CAD build for the part. Positions are in the model's coordinates, mm. A direction names the side the tool comes from. Give positions to 0.01 mm unless a question says otherwise; leave off trailing zeros. Order: outer loops, then holes, each group sorted by start corner. A loop starts at its lowest first (then second) coordinate and runs counter-clockwise, first axis right, second up.
Solid Edge part; units mm, degrees
sketch "Sketch1" plane through (0, 0, 0) normal (0, 0, 1) x (1, 0, 0)
  circle A0 centre (0, 0) radius 15.748
  circle A1 centre (0, 0) radius 7.62
extrude "Protrusion1" add sketch "Sketch1" along normal blind 7.366
sketch "Sketch2" plane through (0, 0, 0) normal (0, 0, 1) x (1, 0, 0)
  circle A0 centre (0, -11.684) radius 6.858
extrude "ExtrudedCutout_1" cut sketch "Sketch2" along normal blind 6.858
sketch "Sketch3" plane through (0, 0, 7.366) normal (0, 0, 1) x (1, 0, 0)
  circle A0 centre (0, -11.684) radius 3.683
extrude "ExtrudedCutout_3" cut sketch "Sketch3" against normal blind 7.0384
pattern_circular "Pattern1" count 4 over 360 about axis through (0, 0, 7.366) along (0, 0, 1) of "ExtrudedCutout_1", "ExtrudedCutout_3"
sketch "Sketch4" plane through (0, 0, 7.366) normal (0, 0, 1) x (1, 0, 0)
  circle A0 centre (0, 0) radius 7.62
  circle A1 centre (-11.684, 0) radius 3.683
  circle A2 centre (0, 11.684) radius 3.683
  circle A3 centre (11.684, 0) radius 3.683
  circle A4 centre (0, -11.684) radius 3.683
  circle A5 centre (0, 0) radius 15.748
extrude "ExtrudedProtrusion_5" add sketch "Sketch4" along normal blind 9.779
sketch "Sketch5" plane through (0, 0, 17.145) normal (0, 0, 1) x (1, 0, 0)
  circle A0 centre (0, 0) radius 19.2555
extrude "ExtrudedCutout_4" cut sketch "Sketch5" against normal blind 6.35
Item 1: Slice it at C-C (x = 5). Give the cut face in (y, z) (3 decimals).
Item 2: Wall check: L1, parallel to X at y = 0, z = 8; L2, parallel to Y at x = -1.5, z = 9.25. Give the ranges that are in metal, low to high.
Item 3: Slice it at A-A (x = 0). Give the cut face in (y, z) (3 decimals), and give its area (3 significant figures).
Item 4: Tool access for faces 1 (the face through (-10.096, 6.672, 3.381)), 2 (the face through (7, 4, 10.795)): list every direction of +Z, -Z, +X, -X, +Y, -Y with a clear straight run to the whole face (end or side of a thin tool).
Item 5: Drop flat-ended pins along their axis: pin 1 Ø8.5 at (x, y) = (0, 11.684) entering from -Z; pin 2 Ø1 at (y, z) = (6.5, 6.5) entering from -X; pin 3 Ø1 at (x, z) = (-11, 4.5) entering from -Y. Give the stop position or say it passes through.
Item 6: Two-plate mould, pull along X, no slides. Class faces 3 (the face through (0.1, 7.8, 6.858)), 4 (the face through (9, 9, 0)): released by +X, released by -X, zero draft, split by the parting line, or undercut.
Item 7: Slice it at D-D (y = -10.5). Give the cut face in (x, z) (1 decimal), and give its area (3 significant figures).
A:
1. outline: (-14.933, 6.858) - (-6.99, 6.858) - (-6.99, 0) - (-5.75, 0) - (-5.75, 10.795) - (-14.933, 10.795) - close; (5.75, 0) - (6.99, 0) - (6.99, 6.858) - (14.933, 6.858) - (14.933, 10.795) - (5.75, 10.795) - close
2. L1: x = -15.75 to -15.37, -8 to -7.62, 7.62 to 8, 15.37 to 15.75
2. L2: y = -15.68 to -15.05, -8.32 to -7.47, 7.47 to 8.32, 15.05 to 15.68
3. outline: (-15.748, 6.858) - (-15.367, 6.858) - (-15.367, 10.795) - (-15.748, 10.795) - close; (-8.001, 6.858) - (-7.62, 6.858) - (-7.62, 10.795) - (-8.001, 10.795) - close; (7.62, 6.858) - (8.001, 6.858) - (8.001, 10.795) - (7.62, 10.795) - close; (15.367, 6.858) - (15.748, 6.858) - (15.748, 10.795) - (15.367, 10.795) - close
3. area: 6.00 mm2
4. face 1: -Z
4. face 2: +Z, +X, -X, +Y, -Y
5. pin 1: stops at z = 6.86
5. pin 2: stops at x = -14.5
5. pin 3: stops at y = -11.74
6. face 3: undercut
6. face 4: zero draft
7. outline: (-11.7, 0) - (-6.8, 0) - (-6.8, 6.9) - (-3.5, 6.9) - (-3.5, 10.8) - (-11.7, 10.8) - close; (3.5, 6.9) - (6.8, 6.9) - (6.8, 0) - (11.7, 0) - (11.7, 10.8) - (3.5, 10.8) - close
7. area: 133 mm2
